Design review of the part built by this model. Coordinates are the model's own, in mm. A direction names the side the tool comes from. Give positions to 0.01 mm unless a question says otherwise; leave off trailing zeros. Loops run counter-clockwise (first coordinate to the right, second up) from the corner with the lowest first, then second, coordinate; pieces in that order, holes last. Notation, with made-up numbers: (-5, -29) -> (37, -29) arc R11 cw to (37, -25) -> close; hole circle Ø4 at (2.5, 9). An arc over 180 degrees is marked (long way). Use CSV: the item, a comma, the result in double quotes. Start each with the question number.
Item 1: We need section D-D (z = -8). State the section outline as (x, y) points (3 decimals).
Item 2: Clearance check with flat-ended pins moving along their axes: pin 1 (9.5 mm diameter, centred on x = 11.11, z = -34.92, fed in from -Y); pin 2 (2.5 mm diameter, centred on x = 4, y = -12.5, fed in from -Z); pin 3 (3 mm diameter, centred on y = -5, z = -8, fed in from +X); pin 4 (11 mm diameter, centred on x = 14.5, z = -22.5, fed in from +Y). State where each tip first meets the part, or that it passes through.
Item 3: For faces 1 (the face through (8.7, -9, -6)), 2 (the face through (18, -9, -4.762)), 3 (the face through (11, -16, -9.208)), list the 3-axis set-ups (+Z, -Z, +X, -X, +Y, -Y) from which the entire face can be reached by the end or side of a thin tool; tool diameter is ignored.
Item 4: The part is to be moulded in two halves that separate along Z. For faces 4 (the face through (4, -9, -4.762)), 5 (the face through (10.868, -25.311, -46.035)), 6 (the face through (22.225, -23, -18)), say which applies: +Z half, -Z half, draft (parallel to the pull), parting line (faces both ways), or undercut.
Item 5: We need section C-C (x = 20). State the section outline as (y, z) points, plus the area to 3 significant figures.
Item 6: Wall thickness on line 1 along Z through (x, y) = (8, -8.5); line 2 along Z through (x, y) = (10, -26.5); line 3 along Z through (x, y) = (8.75, -27.5): over which ranges is each line inside the solid? List them lowest first. Write a range as from..to.
Item 7: We need section B-B (z = -19.5). State the section outline as (x, y) points (3 decimals), plus the area to 3 significant figures.
Item 8: We need section A-A (y = -22.5). State the section outline as (x, z) points (1 decimal), plus the area to 3 significant figures.
from build123d import *

# Parameters (mm, degrees)
F1_DEPTH = 19.05
F3_DEPTH = 12.7
F4_R     = 5.86105
F5_DEPTH = 25.4
F7_DEPTH = 25.4


with BuildPart() as f1:
    # F0 (on Front) → F1 (new body)
    with BuildSketch(Plane.XZ):
        Polygon((22.225, 0), (0, 0), (0, -4.7625), (8.6995, -4.7625), (8.6995, -6.5405), (6.096, -6.5405), (6.096, -9.2075), (16.129, -9.2075), (16.129, -6.5405), (13.5255, -6.5405), (13.5255, -4.7625), (22.225, -4.7625), align=None)
    extrude(amount=F1_DEPTH)

    # F2 (on face) → F3 (join)
    with BuildSketch(Plane.XZ.offset(19.05)):
        with BuildLine():
            Line((8.6995, -4.7625), (0, -4.7625))
            Line((0, -4.7625), (0, -34.925))
            ThreePointArc((0, -34.925), (11.1125, -46.0375), (22.225, -34.925))
            Line((22.225, -34.925), (22.225, -4.7625))
            Line((22.225, -4.7625), (13.5255, -4.7625))
            Line((13.5255, -4.7625), (13.5255, -6.5405))
            Line((13.5255, -6.5405), (16.129, -6.5405))
            Line((16.129, -6.5405), (16.129, -9.2075))
            Line((16.129, -9.2075), (6.096, -9.2075))
            Line((6.096, -9.2075), (6.096, -6.5405))
            Line((6.096, -6.5405), (8.6995, -6.5405))
            Line((8.6995, -6.5405), (8.6995, -4.7625))
        make_face()
        Polygon((22.225, 0), (0, 0), (0, -4.7625), (8.6995, -4.7625), (8.6995, -6.5405), (6.096, -6.5405), (6.096, -9.2075), (16.129, -9.2075), (16.129, -6.5405), (13.5255, -6.5405), (13.5255, -4.7625), (22.225, -4.7625), align=None)
    extrude(amount=F3_DEPTH)

    # F4 (on face) → F5 (cut)
    with BuildSketch(Plane.XZ.offset(31.75)):
        with Locations((11.1125, -34.925)):
            Circle(F4_R)
    extrude(amount=-F5_DEPTH, mode=Mode.SUBTRACT)

    # F6 (on face) → F7 (cut)
    with BuildSketch(Plane.XZ.offset(31.75)):
        with BuildLine():
            Line((17.399, -9.2075), (4.826, -9.2075))
            ThreePointArc((4.826, -9.2075), (1.190625, -14.892203), (4.826, -20.576906))
            Line((4.826, -20.576906), (17.399, -20.576906))
            ThreePointArc((17.399, -20.576906), (21.034375, -14.892203), (17.399, -9.2075))
        make_face()
    extrude(amount=-F7_DEPTH, mode=Mode.SUBTRACT)


solid = f1.part
Results found:
1,outline,"(0, -31.75) -> (22.225, -31.75) -> (22.225, -19.05) -> (16.129, -19.05) -> (16.129, 0) -> (6.096, 0) -> (6.096, -19.05) -> (0, -19.05) -> close"
2,pin 1,"through"
2,pin 2,"z = -4.76"
2,pin 3,"x = 16.13"
2,pin 4,"y = -19.05"
3,face 1,"-X, +Y"
3,face 2,"+X, +Y"
3,face 3,"+Y, -Y"
4,face 4,"undercut"
4,face 5,"-Z half"
4,face 6,"draft"
5,outline,"(-31.75, -41.6) -> (-19.05, -41.6) -> (-19.05, -18.34) -> (-31.75, -18.34) -> close; (-31.75, -11.44) -> (-19.05, -11.44) -> (-19.05, -4.76) -> (0, -4.76) -> (0, 0) -> (-31.75, 0) -> close"
5,area,"531 mm²"
6,line 1,"-9.21..-6.54, -4.76..0"
6,line 2,"-45.98..-40.68, -29.17..-20.58, -9.21..0"
6,line 3,"-45.78..-40.29, -29.56..-20.58, -9.21..0"
7,outline,"(0, -31.75) -> (3.212, -31.75) -> (3.212, -19.05) -> (0, -19.05) -> close; (19.013, -31.75) -> (22.225, -31.75) -> (22.225, -19.05) -> (19.013, -19.05) -> close"
7,area,"81.6 mm²"
8,outline,"(0, -34.9) arc R11.1 ccw to (22.2, -34.9) -> (22.2, 0) -> (0, 0) -> close; hole (4.8, -20.6) -> (17.4, -20.6) arc R6.3 ccw to (17.4, -9.2) -> (4.8, -9.2) arc R6.3 ccw to start; hole circle Ø11.7 at (11.1, -34.9)"
8,area,"660 mm²"
